Autodesk Inventor part; units mm, degrees
ref_plane "YZ Plane" through (0, 0, 0) normal (1, 0, 0) x (0, 1, 0)
ref_plane "XZ Plane" through (0, 0, 0) normal (0, 1, 0) x (-1, 0, 0)
ref_plane "XY Plane" through (0, 0, 0) normal (0, 0, 1) x (1, 0, 0)
sketch "スケッチ1" plane through (0, 0, 0) normal (0, 1, 0) x (-1, 0, 0)
  line L0 (1.7293, 44.1636) -> (-1.2707, 44.1636)
  line L1 (-1.2707, 44.1636) -> (-1.2707, -5.8364)
  line L2 (-1.2707, -5.8364) -> (1.7293, -5.8364)
  line L3 (1.7293, -5.8364) -> (1.7293, 44.1636)
  line L4 (31.7293, -2.8364) -> (1.7293, -2.8364)
  line L5 (1.7293, -2.8364) -> (1.7293, -5.8364)
  line L6 (1.7293, -5.8364) -> (31.7293, -5.8364)
  line L7 (31.7293, -5.8364) -> (31.7293, -2.8364)
  line L8 (31.7293, -5.8364) -> (28.7293, -5.8364)
  line L9 (28.7293, -5.8364) -> (28.7293, -51.7922)
  line L10 (28.7293, -51.7922) -> (31.7293, -51.7922)
  line L11 (31.7293, -51.7922) -> (31.7293, -5.8364)
  point P0 (0, 0)
  dimension "d0" = 3
  dimension "d1" = 50
  dimension "d2" = 30
  dimension "d3" = 3
  dimension "d4" = 3
extrude "押し出し1" add sketch "スケッチ1" along normal blind 20
properties part number "recreat1"
The model under review builds one solid part; all positions refer to its coordinate system, in mm. A direction names the side the tool comes from. Round coordinates to 2 decimals unless told otherwise and drop trailing zeros. Order: outer loops, then holes, each group sorted by start corner. A loop starts at its lowest first (then second) coordinate and runs counter-clockwise, first axis right, second up.
(1) Take a section at B-B, the plane z = -31. State the section outline as (x, y) points.
Working result:
outline: (-31.73, 0) - (-28.73, 0) - (-28.73, 20) - (-31.73, 20) - close
(2) Wall thickness on L1, parallel to X at y = 10.75, z = -14; L2, parallel to Z at x = -29, y = 14.5; L3, parallel to Z at x = -9.5, y = 3.5: over which ranges is each line inside the solid? List them lowest first.
Working result:
L1: x = -31.73 to -28.73
L2: z = -51.79 to -2.84
L3: z = -5.84 to -2.84
(3) Take a section at A-A, the plane y = 10. State the section outline as (x, z) points.
Working result:
outline: (-31.73, -51.79) - (-28.73, -51.79) - (-28.73, -5.84) - (1.27, -5.84) - (1.27, 44.16) - (-1.73, 44.16) - (-1.73, -2.84) - (-31.73, -2.84) - close
(4) For P1, Ø12, axis at x = -20.5, y = 12, coming from the -Z side; P2, Ø5, axis at x = -22.5, y = 12.5, coming from the +Z side; P3, Ø10, axis at y = 9, z = 10, coming from the -X side, all flat-tipped, find the tip position at first contact; note any pin that passes through.
Working result:
P1: stops at z = -5.84
P2: stops at z = -2.84
P3: stops at x = -1.73
(5) Take a section at C-C, the plane x = -4. State the section outline as (y, z) points, plus the area to 3 significant figures.
Working result:
outline: (0, -5.84) - (20, -5.84) - (20, -2.84) - (0, -2.84) - close
area: 60.0 mm2
(6) Tool access review of faces 1 (the face through (-1.729, 10, 20)), 2 (the face through (-28.729, 10, -28)), 3 (the face through (-13, 0, -4)): name each direction out of +Z, -Z, +X, -X, +Y, -Y from which nothing blocks a thin tool from reaching the whole face with its end or side.
Working result:
face 1: +Z, -X, +Y, -Y
face 2: -Z, +X, +Y, -Y
face 3: +Z, -Z, +X, -X, -Y
